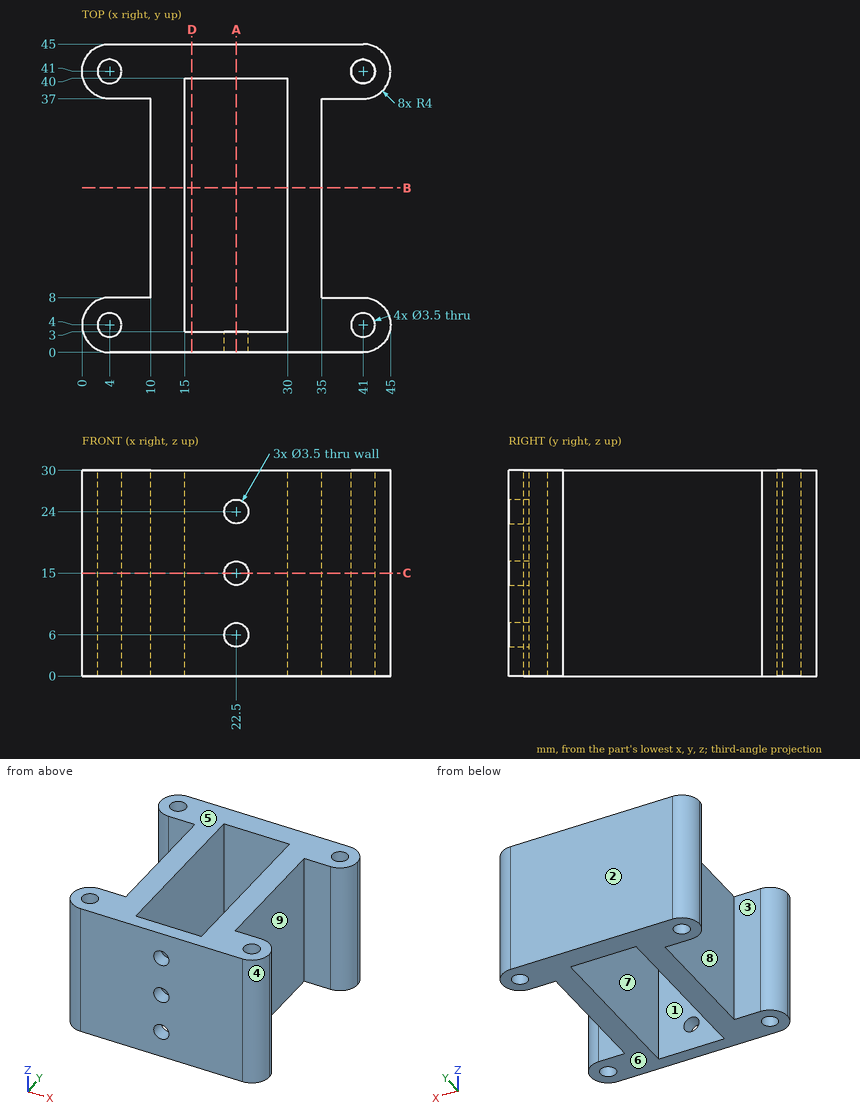
Could you check a few things on this drawing? It's one solid part, dimensions in mm from its lowest x, y, z. A direction names the side the tool comes from. Give positions to 0.01 mm unless a question says otherwise; leave off trailing zeros. Loops run counter-clockwise (first coordinate to the right, second up) from the corner with the lowest first, then second, coordinate; pieces in that order, holes last. Notation, with made-up numbers: (-1, 31.25) -> (10, 31.25) arc R15 cw to (10, 49.25) -> close; hole circle Ø8 at (-16.5, 0.25). An arc over 180 degrees is marked (long way). Use one line per item in the form item = value. Start each with the question number.
1) Imagine slicing it at B-B (y = 24). Please give me the cut outline in (x, z), then the cut area to 3 significant figures.
2) Thinking about a two-plate mould opening in Y: for the marked faces 1, 2, 3 and 4, which applies, +Y half, -Y half, draft (parallel to the pull), parting line (faces both ways), or undercut?
3) Imagine slicing it at D-D (x = 16). Please give me the cut outline in (y, z), then the cut area to 3 significant figures.
4) For P1, Ø5, axis at y = 30, z = 9, coming from the -X side; P2, Ø2, axis at y = 31.5, z = 26.5, coming from the +X side, each with a flat end and sliding along its axis, tell me the tip position at first contact or that it passes through.
5) Imagine slicing it at C-C (z = 15). Count the separate pieces of the cut face and the enclosed holes in it.
6) Please list where these lines run through material, in increasing order: line 1 along Y through (x, z) = (4, 14.75); line 2 along Y through (x, z) = (7.5, 22.5); line 3 along X through (y, z) = (12, 23.75).
7) Imagine slicing it at A-A (x = 22.5). Please give me the cut outline in (y, z), then the cut area to 4 significant figures.
8) Which directions (+Z, -Z, +X, -X, +Y, -Y) give clear straight access to the entire face, cutting with the end or side of a thin tool? Please do the marked faces 5, 6, 7, 8 and 9.
Check values:
q1.outline = (10, 0) -> (15, 0) -> (15, 30) -> (10, 30) -> close; (30, 0) -> (35, 0) -> (35, 30) -> (30, 30) -> close
q1.area = 300 mm^2
q2.face_1 = undercut
q2.face_2 = +Y half
q2.face_3 = undercut
q2.face_4 = -Y half
q3.outline = (0, 0) -> (3, 0) -> (3, 30) -> (0, 30) -> close; (40, 0) -> (45, 0) -> (45, 30) -> (40, 30) -> close
q3.area = 240 mm^2
q4.P1 = 10
q4.P2 = 35
q5.separate_pieces = 1
q5.enclosed_holes = 4
q6.line_1 = 0 to 2.25, 5.75 to 8, 37 to 39.25, 42.75 to 45
q6.line_2 = 0 to 8, 37 to 45
q6.line_3 = 10 to 15, 30 to 35
q7.outline = (0, 0) -> (3, 0) -> (3, 4.25) -> (0, 4.25) -> close; (0, 7.75) -> (3, 7.75) -> (3, 13.25) -> (0, 13.25) -> close; (0, 16.75) -> (3, 16.75) -> (3, 22.25) -> (0, 22.25) -> close; (0, 25.75) -> (3, 25.75) -> (3, 30) -> (0, 30) -> close; (40, 0) -> (45, 0) -> (45, 30) -> (40, 30) -> close
q7.area = 208.5 mm^2
q8.face_5 = +Z, +X, -X, +Y, -Y
q8.face_6 = -Z, +X, -X, +Y, -Y
q8.face_7 = +Z, -Z
q8.face_8 = +Z, -Z, -X
q8.face_9 = +Z, -Z, +X
